Verification items for the finished model (mm, model axes). A direction names the side the tool comes from. Round coordinates to 2 decimals unless told otherwise and drop trailing zeros. Order: outer loops, then holes, each group sorted by start corner. A loop starts at its lowest first (then second) coordinate and runs counter-clockwise, first axis right, second up. Notation, with made-up numbers: (68, -5) -> (125, -5) arc R29 ccw to (125, 22) -> close; hole circle Ø10 at (1, -19). An arc over 180 degrees is marked (long way). Return JSON: item names as keys, results as strings. Group by question number.
Item 1: Sectioned sample at B-B on y = 7. Record the cut outline in (x, z) (3 decimals).
Item 2: Scan lines: probe 1 along X at (y, z) = (4, -19.05) (3 decimals); probe 2 along X at (y, z) = (7, 19.05) (3 decimals); probe 3 along Y at (x, z) = (-16.5, -11). Record each from-to range of solid material in increasing order. Write a range as from..to.
Item 3: Sectioned sample at D-D on z = 0. Record the cut outline in (x, y).
Item 4: Sectioned sample at A-A on x = -31.75. Record the cut outline in (y, z) (3 decimals), plus the area to 3 significant figures.
Item 5: Depth check by flat-ended pin: pin 1 Ø8.5 at (x, z) = (-31.75, 19.05) entering from +Y; pin 2 Ø10.5 at (x, z) = (31.75, -19.05) entering from -Y; pin 3 Ø6 at (y, z) = (43.5, 3) entering from -X; pin 4 Ø5 at (x, y) = (-13, 19.5) entering from -Z. Enter the tip coordinate at first touch or a pass-through.
Item 6: Draft check along X on faces 3 (the flat face through (9, 12.7, -15)), 4 (the cylindrical face through (-34.85, 6.26, -19.74)), 5 (the flat face through (44.45, 6, 0)), 6 (the cylindrical face through (35.07, 6.26, -19.49)). Enter one of: pulls with the +X half, pulls with the -X half, needs draft (parallel to the pull), parting line crosses it, or undercut.
Item 7: Access from +Z, -Z, +X, -X, +Y, -Y to the whole of each face (thin tool, end or side, straight path). Record for faces 1 (the flat face through (-1, 6, -31.75)), 2 (the cylindrical face through (7.7, 33.4, 10.1)).
Item 8: Sectioned sample at C-C on z = -19.05. Record the cut outline in (x, y) (3 decimals), plus the area to 3 significant figures.
```python
from build123d import *

# Parameters (mm, degrees)
SKETCH1_W           = 88.9
SKETCH1_H           = 63.5
SKETCH1_R           = 3.175
SKETCH1_R_2         = 3.349234597
BOSS_EXTRUDE1_DEPTH = 12.7
SKETCH2_R           = 12.7
BOSS_EXTRUDE2_DEPTH = 38.1
CHAMFER1_SIZE       = 3.81


with BuildPart() as part:
    # Sketch1 → Boss-Extrude1 (new body)
    with BuildSketch(Plane(origin=(0, 0, 0), x_dir=(1, 0, 0), z_dir=(0, 1, 0))):
        Rectangle(SKETCH1_W, SKETCH1_H)
        with Locations(Location((-31.75, 19.05, 0), (0, 0, 270))):
            Circle(SKETCH1_R, mode=Mode.SUBTRACT)
        with Locations(Location((-31.75, -19.05, 0), (0, 0, 270))):
            Circle(SKETCH1_R, mode=Mode.SUBTRACT)
        with Locations(Location((31.75, -19.05, 0), (0, 0, 270))):
            Circle(SKETCH1_R, mode=Mode.SUBTRACT)
        with Locations(Location((31.75, 19.05, 0), (0, 0, 270))):
            Circle(SKETCH1_R_2, mode=Mode.SUBTRACT)
    extrude(amount=BOSS_EXTRUDE1_DEPTH)

    # Sketch2 → Boss-Extrude2 (add)
    with BuildSketch(Plane(origin=(0, 12.7, 0), x_dir=(1, 0, 0), z_dir=(0, 1, 0))):
        with Locations(Location((0, 0, 0), (0, 0, 90))):
            Circle(SKETCH2_R)
    extrude(amount=BOSS_EXTRUDE2_DEPTH)

    # Chamfer1
    chamfer1_edges = [part.edges().sort_by_distance(p)[0] for p in [
        (0, 12.7, 12.7),
    ]]
    chamfer(chamfer1_edges, length=CHAMFER1_SIZE)


solid = part.part
```
Recorded:
{
 "1": {"outline": "(-44.45, -31.75) -> (44.45, -31.75) -> (44.45, 31.75) -> (-44.45, 31.75) -> close; hole circle Ø6.35 at (-31.75, -19.05); hole circle Ø6.35 at (-31.75, 19.05); hole circle Ø6.698 at (31.75, -19.05); hole circle Ø6.35 at (31.75, 19.05)"},
 "2": {"probe 1": "-44.45..-34.925, -28.575..28.401, 35.099..44.45", "probe 2": "-44.45..-34.925, -28.575..28.575, 34.925..44.45", "probe 3": "0..12.7"},
 "3": {"outline": "(-44.45, 0) -> (44.45, 0) -> (44.45, 12.7) -> (16.51, 12.7) -> (12.7, 16.51) -> (12.7, 50.8) -> (-12.7, 50.8) -> (-12.7, 16.51) -> (-16.51, 12.7) -> (-44.45, 12.7) -> close"},
 "4": {"outline": "(0, -31.75) -> (12.7, -31.75) -> (12.7, -22.225) -> (0, -22.225) -> close; (0, -15.875) -> (12.7, -15.875) -> (12.7, 15.875) -> (0, 15.875) -> close; (0, 22.225) -> (12.7, 22.225) -> (12.7, 31.75) -> (0, 31.75) -> close", "area": "645 mm²"},
 "5": {"pin 1": "y = 12.7", "pin 2": "y = 0", "pin 3": "x = -12.7", "pin 4": "z = -7.14"},
 "6": {"face 3": "needs draft", "face 4": "undercut", "face 5": "pulls with the +X half", "face 6": "undercut"},
 "7": {"face 1": "-Z, +X, -X, +Y, -Y", "face 2": "+Y"},
 "8": {"outline": "(-44.45, 0) -> (-34.925, 0) -> (-34.925, 12.7) -> (-44.45, 12.7) -> close; (-28.575, 0) -> (28.401, 0) -> (28.401, 12.7) -> (-28.575, 12.7) -> close; (35.099, 0) -> (44.45, 0) -> (44.45, 12.7) -> (35.099, 12.7) -> close", "area": "963 mm²"}
}
